```python
from build123d import *

# Parameters (mm, degrees)
BOSS_EXTRUDE1_DEPTH = 459.74
SKETCH3_W           = 117.668752198
SKETCH3_H           = 459.74
CUT_EXTRUDE1_DEPTH  = 10
SKETCH4_W           = 9.725175386
SKETCH4_H           = 183.54
SKETCH4_H_2         = 200
CUT_EXTRUDE3_DEPTH  = 63


with BuildPart() as part:
    # Sketch1 → Boss-Extrude1 (new body)
    with BuildSketch(Plane.XY):
        Polygon((358.121789204, 754.380000017), (137.961261276, 754.380000017), (137.961261276, 744.380000017), (562.803601281, 744.380000017), (562.803601281, 754.380000017), align=None)
    extrude(amount=BOSS_EXTRUDE1_DEPTH)

    # Sketch3 → Cut-Extrude1 (cut)
    with BuildSketch(Plane.XZ.offset(-744.380000017)):
        with Locations((196.795637375, 229.87)):
            Rectangle(SKETCH3_W, SKETCH3_H)
    extrude(amount=-CUT_EXTRUDE1_DEPTH, mode=Mode.SUBTRACT)

    # Sketch4 → Cut-Extrude3 (cut)
    with BuildSketch(Plane(origin=(0, 754.380000017, 0), x_dir=(1, 0, 0), z_dir=(0, 1, 0))):
        with Locations((260.492601167, -367.97)):
            Rectangle(SKETCH4_W, SKETCH4_H)
        with Locations((260.492601167, -100)):
            Rectangle(SKETCH4_W, SKETCH4_H_2)
        with BuildLine():
            Line((333.464234552, -459.74), (369.761877542, -561.839328351))
            Line((369.761877542, -561.839328351), (604.247212907, -525.668487146))
            Line((604.247212907, -525.668487146), (681.481358703, 161.10923172))
            Line((681.481358703, 161.10923172), (358.740146189, 101.846462791))
            Line((358.740146189, 101.846462791), (383.521789204, 0))
            ThreePointArc((383.521789204, 0), (437.403325931, -22.318463274), (459.721789204, -76.2))
            Line((459.721789204, -76.2), (460.501916297, -459.74))
            Line((460.501916297, -459.74), (409.216807378, -459.74))
            Line((409.216807378, -459.74), (408.921789204, -449.58))
            Line((408.921789204, -449.58), (332.721789204, -449.58))
            Line((332.721789204, -449.58), (333.464234552, -459.74))
        make_face()
    extrude(amount=-CUT_EXTRUDE3_DEPTH, mode=Mode.SUBTRACT)


solid = part.part
```
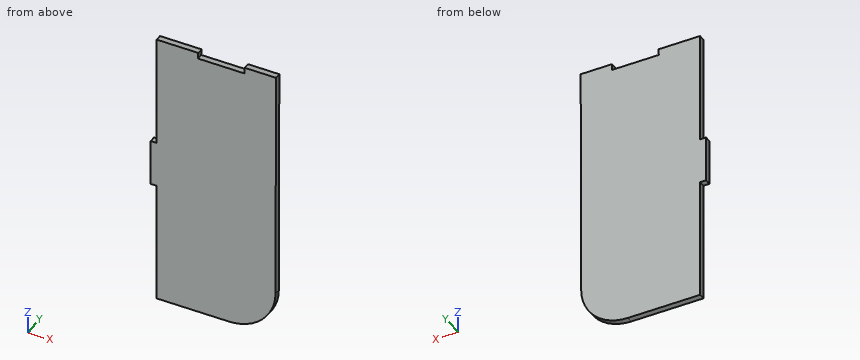
Verification items for the finished model (mm, model axes). Give positions to 0.01 mm unless a question says otherwise; leave off trailing zeros. Loops run counter-clockwise (first coordinate to the right, second up) from the corner with the lowest first, then second, coordinate; pieces in that order, holes last.
1. Section check B-B, the plane z = 391.5. Enter the section's corners in (x, y), then the cut area to 3 significant figures.
2. Thickness scan on line 1 (X direction, y = 747.5, z = 112); line 2 (Z direction, x = 377.5, y = 753.5); line 3 (Z direction, x = 414, y = 751). Record the ranges inside material, lowest first.
3. Section check C-C, the plane x = 362. Enter the section's corners in (y, z), then the cut area to 3 significant figures.
4. Section check A-A, the plane y = 751.5. Enter the section's corners in (x, z), then the cut area to 3 significant figures.
5. Go/stop test with flat-tipped pins: pin 1 Ø2 at (y, z) = (749, 294) entering from -X; pin 2 Ø3 at (x, y) = (260.5, 749) entering from -Z. Record where each tip stops, or that it passes through.
Geometry says:
1. outline: (265.36, 744.38) - (460.36, 744.38) - (460.36, 754.38) - (265.36, 754.38) - close
1. area: 1,950 mm2
2. line 1: x = 265.36 to 459.79
2. line 2: z = 0 to 449.58
2. line 3: z = 6.36 to 459.74
3. outline: (744.38, 0) - (754.38, 0) - (754.38, 449.58) - (744.38, 449.58) - close
3. area: 4,500 mm2
4. outline: (255.63, 200) - (265.36, 200) - (265.36, 0) - (383.52, 0) arc R76.2 ccw to (459.72, 76.2) - (460.5, 459.74) - (409.22, 459.74) - (408.92, 449.58) - (332.72, 449.58) - (333.46, 459.74) - (265.36, 459.74) - (265.36, 276.2) - (255.63, 276.2) - close
4. area: 88,200 mm2
5. pin 1: stops at x = 265.36
5. pin 2: stops at z = 200
